Check sheet for the drawn part. Datum: minimum x, y, z corner. Units: mm. A direction names the side the tool comes from. Coordinates: 2 decimals unless noted, no trailing zeros. Order: outer loops, then holes, each group sorted by start corner. A loop starts at its lowest first (then second) coordinate and runs counter-clockwise, first axis right, second up. Notation, with made-up numbers: (36.5, -9) - (76.5, -9) arc R21 cw to (76.5, 15) - close; hole circle Ø5 at (47.25, 84.25). An arc over 180 degrees is marked (long way). Return JSON: item names as keys, results as strings. Group by question number.
Item 1: Section check B-B on z = 12.25. Enter the section's corners in (x, y), then the cut area to 3 significant figures.
Item 2: Section check D-D on y = 1.1. Enter the section's corners in (x, z), then the cut area to 3 significant figures.
Item 3: Section check C-C on z = 3.5. Enter the section's corners in (x, y), then the cut area to 3 significant figures.
Item 4: Scan lines: probe 1 along Z at (x, y) = (12.25, 1.6); probe 2 along X at (y, z) = (2.35, 12.25); probe 3 along Y at (x, z) = (10.25, 5.25). Record each from-to range of solid material in increasing order.
Item 5: Draft check along Z on the marked faces 1, 2 and 3. Enter one of: pulls with the +Z half, pulls with the -Z half, needs draft (parallel to the pull), parting line crosses it, or undercut.
Item 6: Tool access check on the marked faces 4 and 5. Record the directions out of +Z, -Z, +X, -X, +Y, -Y that give a thin tool (end or side, any length) a straight path to the whole face; none if there is none.
Item 7: Gauge pin test, flat ends, axial feed: pin 1 (3 mm diameter, centred on x = 6, y = 4, fed in from +Z); pin 2 (1.5 mm diameter, centred on x = 13, z = 4.5, fed in from +Y); pin 3 (3 mm diameter, centred on x = 12.25, z = 4.25, fed in from -Y); pin 4 (2 mm diameter, centred on x = 21.5, y = 1.5, fed in from +Z). Record the tip position at first contact, or that the pin passes through.
Item 8: Section check A-A on x = 12.25. Enter the section's corners in (y, z), then the cut area to 3 significant figures.
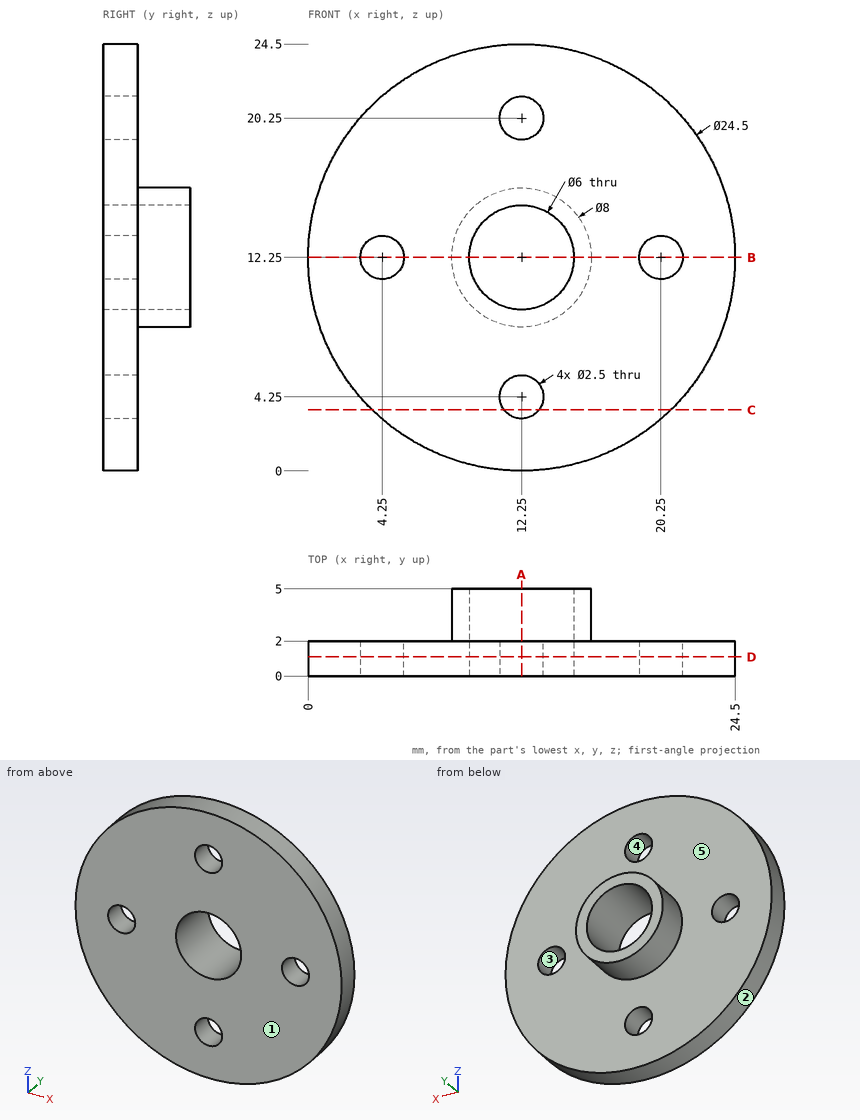
Computed:
{
 "1": {"outline": "(0, 0) - (3, 0) - (3, 2) - (0, 2) - close; (5.5, 0) - (9.25, 0) - (9.25, 5) - (8.25, 5) - (8.25, 2) - (5.5, 2) - close; (15.25, 0) - (19, 0) - (19, 2) - (16.25, 2) - (16.25, 5) - (15.25, 5) - close; (21.5, 0) - (24.5, 0) - (24.5, 2) - (21.5, 2) - close", "area": "33.0 mm²"},
 "2": {"outline": "circle Ø24.5 at (12.25, 12.25); hole circle Ø2.5 at (4.25, 12.25); hole circle Ø6 at (12.25, 12.25); hole circle Ø2.5 at (12.25, 4.25); hole circle Ø2.5 at (12.25, 20.25); hole circle Ø2.5 at (20.25, 12.25)", "area": "424 mm²"},
 "3": {"outline": "(3.68, 0) - (11.25, 0) - (11.25, 2) - (3.68, 2) - close; (13.25, 0) - (20.82, 0) - (20.82, 2) - (13.25, 2) - close", "area": "30.3 mm²"},
 "4": {"probe 1": "z = 0 to 3, 5.5 to 9.25, 15.25 to 19, 21.5 to 24.5", "probe 2": "x = 8.25 to 9.25, 15.25 to 16.25", "probe 3": "y = 0 to 2"},
 "5": {"face 1": "needs draft", "face 2": "parting line crosses it", "face 3": "undercut"},
 "6": {"face 4": "+Y, -Y", "face 5": "+Y"},
 "7": {"pin 1": "passes through", "pin 2": "stops at y = 2", "pin 3": "stops at y = 0", "pin 4": "stops at z = 21.31"},
 "8": {"outline": "(0, 0) - (2, 0) - (2, 3) - (0, 3) - close; (0, 5.5) - (2, 5.5) - (2, 8.25) - (5, 8.25) - (5, 9.25) - (0, 9.25) - close; (0, 15.25) - (5, 15.25) - (5, 16.25) - (2, 16.25) - (2, 19) - (0, 19) - close; (0, 21.5) - (2, 21.5) - (2, 24.5) - (0, 24.5) - close", "area": "33.0 mm²"}
}
